```python
from build123d import *

# Parameters (mm, degrees)
ESQUISSE1_W                  = 38
ESQUISSE1_H                  = 38
BOSS_EXTRU_1_DEPTH           = 1.6
CONG_1_R                     = 1
ESQUISSE2_R                  = 1
ENL_V_MAT_EXTRU_1_DEPTH      = 2.6
ESQUISSE3_R                  = 1
ENL_V_MAT_EXTRU_2_DEPTH      = 2.6
R_P_TITION_CIRCULAIRE1_COUNT = 4
ESQUISSE4_W                  = 17
ESQUISSE4_H                  = 4.5
BOSS_EXTRU_2_DEPTH           = 2


with BuildPart() as part:
    # Esquisse1 → Boss.-Extru.1 (new body)
    with BuildSketch(Plane(origin=(0, 0, 0), x_dir=(0, 0, -1), z_dir=(1, 0, 0))):
        Rectangle(ESQUISSE1_W, ESQUISSE1_H)
    extrude(amount=BOSS_EXTRU_1_DEPTH)

    # Cong_1
    cong_1_edges = [part.edges().sort_by_distance(p)[0] for p in [
        (0.8, 19, 19),
        (0.8, 19, -19),
        (0.8, -19, -19),
        (0.8, -19, 19),
    ]]
    fillet(cong_1_edges, radius=CONG_1_R)

    # Esquisse2 → Enl_v. mat.-Extru.1 (cut, through all)
    with BuildSketch(Plane(origin=(1.6, 0, 0), x_dir=(0, 0, -1), z_dir=(1, 0, 0))):
        with Locations((-10, 0)):
            Circle(ESQUISSE2_R)
        with Locations((10, 0)):
            Circle(ESQUISSE2_R)
    extrude(amount=-ENL_V_MAT_EXTRU_1_DEPTH, mode=Mode.SUBTRACT)

    # Esquisse3 → Enl_v. mat.-Extru.2 (cut, through all)
    with BuildSketch(Plane(origin=(1.6, 0, 0), x_dir=(0, 0, -1), z_dir=(1, 0, 0))):
        with Locations((16.970562748, 16.970562748)):
            Circle(ESQUISSE3_R)
        with BuildLine():
            Line((13.611805538, 15.379572491), (13.965358928, 15.733125881))
            ThreePointArc((13.965358928, 15.733125881), (15.733125881, 15.733125881), (15.733125881, 13.965358928))
            Line((15.733125881, 13.965358928), (15.379572491, 13.611805538))
            ThreePointArc((15.379572491, 13.611805538), (13.611805538, 13.611805538), (13.611805538, 15.379572491))
        make_face()
    enl_v_mat_extru_2 = extrude(amount=-ENL_V_MAT_EXTRU_2_DEPTH, mode=Mode.SUBTRACT)

    # R_p_tition circulaire1: Enl_v. mat.-Extru.2 ×4 about axis
    r_p_tition_circulaire1_axis = Axis((0, 0, 0), (1, 0, 0))
    for i in range(1, R_P_TITION_CIRCULAIRE1_COUNT):
        add(enl_v_mat_extru_2.rotate(r_p_tition_circulaire1_axis, i * 360 / R_P_TITION_CIRCULAIRE1_COUNT), mode=Mode.SUBTRACT)

    # Esquisse4 → Boss.-Extru.2 (add)
    with BuildSketch(Plane(origin=(1.6, 0, 0), x_dir=(0, 0, -1), z_dir=(1, 0, 0))):
        with Locations((0, -15.75)):
            Rectangle(ESQUISSE4_W, ESQUISSE4_H)
    extrude(amount=BOSS_EXTRU_2_DEPTH)


solid = part.part
```
Input: part model. Units: mm. Frame: model coordinates. A direction names the side the tool comes from. Give positions to 0.01 mm unless a question says otherwise; leave off trailing zeros. Order: outer loops, then holes, each group sorted by start corner. A loop starts at its lowest first (then second) coordinate and runs counter-clockwise, first axis right, second up. Notation, with made-up numbers: (-1, 84.5) -> (49, 84.5) arc R34 cw to (49, 114.5) -> close; hole circle Ø7 at (20.25, 88). An arc over 180 degrees is marked (long way). Write each question's results on one line, items separated by ' | '. Start each with the question number.
Item 1: Mould query, pull axis Z, two halves, no side actions, for faces 1 (the flat face through (1, 0, 19)), 2 (the flat face through (3, -18, 0)), 3 (the cylindrical face through (0.8, 16.6, -17.9)), 4 (the cylindrical face through (0.8, -16.6, 17.9)). Classes: pulls with the +Z half, pulls with the -Z half, needs draft (parallel to the pull), parting line crosses it, or undercut.
Item 2: Line query: line 1 (Z direction, x = 0.65, y = -15.5); line 2 (Y direction, x = 0.25, z = -15); line 3 (X direction, y = -6, z = 15). Output: solid intervals per line, ascending.
Item 3: Cut plane C-C on z = 4.5. Return the cut outline in (x, y).
Item 4: Cut plane B-B on z = 10. Return the cut outline in (x, y).
Item 5: Contact query for flat-ended pins moving along their axis: P1, Ø3, axis at y = 16.97, z = 16.97, coming from the -X side; P2, Ø0.6, axis at x = 2.5, z = 3.5, coming from the +Y side; P3, Ø0.6, axis at x = 2.5, z = -4, coming from the -Y side; P4, Ø8, axis at y = 8, z = 14, coming from the +X side. Output: stop coordinate, or through.
Item 6: Cut plane A-A on y = 0. Return the cut outline in (x, z).
Item 7: Cut plane D-D on y = -6. Return the cut outline in (x, z).
Item 8: Set-up query: faces 5 (the cylindrical face through (0.811, -18.699, 18.715)), 6 (the flat face through (3, -16, 8.5)). Return all of +Z, -Z, +X, -X, +Y, -Y with unobstructed straight access to the full face (end or side cutting, diameter ignored); none if empty.
Established:
1) face 1: pulls with the +Z half | face 2: needs draft | face 3: undercut | face 4: undercut
2) line 1: -19 to -15.92, -13.73 to 13.73, 15.92 to 19 | line 2: -19 to -16.09, -13.35 to 13.35, 16.09 to 19 | line 3: 0 to 1.6
3) outline: (0, -19) -> (1.6, -19) -> (1.6, -18) -> (3.6, -18) -> (3.6, -13.5) -> (1.6, -13.5) -> (1.6, 19) -> (0, 19) -> close
4) outline: (0, -19) -> (1.6, -19) -> (1.6, -1) -> (0, -1) -> close; (0, 1) -> (1.6, 1) -> (1.6, 19) -> (0, 19) -> close
5) P1: x = 0 | P2: y = -13.5 | P3: y = -18 | P4: x = 1.6
6) outline: (0, -19) -> (1.6, -19) -> (1.6, -11) -> (0, -11) -> close; (0, -9) -> (1.6, -9) -> (1.6, 9) -> (0, 9) -> close; (0, 11) -> (1.6, 11) -> (1.6, 19) -> (0, 19) -> close
7) outline: (0, -19) -> (1.6, -19) -> (1.6, 19) -> (0, 19) -> close
8) face 5: +Z, +X, -X, -Y | face 6: +Z, +X, +Y, -Y
